Verification items for the finished model (mm, model axes). A direction names the side the tool comes from. Round coordinates to 2 decimals unless told otherwise and drop trailing zeros. Order: outer loops, then holes, each group sorted by start corner. A loop starts at its lowest first (then second) coordinate and runs counter-clockwise, first axis right, second up. Notation, with made-up numbers: M 0,76.25 L 21,76.25 A31 cw 21,113.25 Z; hole C -28,21 d3. An arc over 180 degrees is marked long. Answer as a JSON object with one key per item and string values. Group by question number.
```python
from build123d import *

# Parameters (mm, degrees)
SKETCH1_R           = 5.55
BOSS_EXTRUDE1_DEPTH = 29.62
CHAMFER1_SIZE       = 2.38
CHAMFER1_SIZE2      = 3.175
SKETCH2_R           = 2
BOSS_EXTRUDE2_DEPTH = 48
SKETCH3_R           = 0.43
BOSS_EXTRUDE3_DEPTH = 35


with BuildPart() as part:
    # Sketch1 → Boss-Extrude1 (new body)
    with BuildSketch(Plane(origin=(0, 0, 0), x_dir=(1, 0, 0), z_dir=(0, 1, 0))):
        Circle(SKETCH1_R)
    extrude(amount=BOSS_EXTRUDE1_DEPTH)

    # Chamfer1
    chamfer1_edges = [part.edges().sort_by_distance(p)[0] for p in [
        (-5.55, 29.62, 0),
    ]]
    chamfer1_side = [part.faces().sort_by_distance(p)[0] for p in [
        (-5.55, 14.81, 0),
    ]]
    chamfer(chamfer1_edges, length=CHAMFER1_SIZE, length2=CHAMFER1_SIZE2, reference=chamfer1_side[0])

    # Sketch2 → Boss-Extrude2 (add)
    with BuildSketch(Plane(origin=(0, 29.62, 0), x_dir=(1, 0, 0), z_dir=(0, 1, 0))):
        Circle(SKETCH2_R)
    extrude(amount=BOSS_EXTRUDE2_DEPTH)

    # Sketch3 → Boss-Extrude3 (add)
    with BuildSketch(Plane(origin=(0, 77.62, 0), x_dir=(1, 0, 0), z_dir=(0, 1, 0))):
        with Locations((0, 1.143312096)):
            Circle(SKETCH3_R)
    extrude(amount=BOSS_EXTRUDE3_DEPTH)


solid = part.part
```
Q1. Tool access check on faces 1 (the face through (2.98, 13.43, -4.68)), 2 (the face through (0, 53, 2)). Record the directions out of +Z, -Z, +X, -X, +Y, -Y that give a thin tool (end or side, any length) a straight path to the whole face; none if there is none.
Q2. Thickness scan on line 1 (Y direction, x = 0.25, z = 0); line 2 (Y direction, x = -1.75, z = -1.25); line 3 (X direction, y = 27, z = -0.5). Record the ranges inside material, lowest first. Write a range as from..to.
Q3. Gauge pin test, flat ends, axial feed: pin 1 Ø4 at (y, z) = (36.5, 1) entering from +X; pin 2 Ø2 at (y, z) = (61, 4) entering from +X; pin 3 Ø3 at (x, y) = (1, 81.5) entering from -Z; pin 4 Ø1.2 at (x, z) = (0, 0) entering from +Y. Record the tip position at first contact, or that the pin passes through.
Q4. Cross-section at A-A, the plane y = 54. Record the cut outline in (x, z).
Conclusion:
{
 "1": {"face 1": "+Y, -Y", "face 2": "+Y"},
 "2": {"line 1": "0..77.62", "line 2": "0..29.62", "line 3": "-5.53..5.53"},
 "3": {"pin 1": "x = 2", "pin 2": "through", "pin 3": "z = -1.57", "pin 4": "y = 77.62"},
 "4": {"outline": "C 0,0 d4"}
}
